Source: CAD feature listing. Evaluate the final solid. Frame: model axes, mm. Face numbers are marked on the shaded views. Round coordinates to 2 decimals unless told otherwise and drop trailing zeros. Order: outer loops, then holes, each group sorted by start corner. A loop starts at its lowest first (then second) coordinate and runs counter-clockwise, first axis right, second up. Notation, with made-up numbers: (76, -22.75) -> (86, -22.75) arc R20 cw to (86, 12.25) -> close; hole circle Ø3 at (87, 26). An arc over 180 degrees is marked (long way). Answer as CSV lines item,"result".
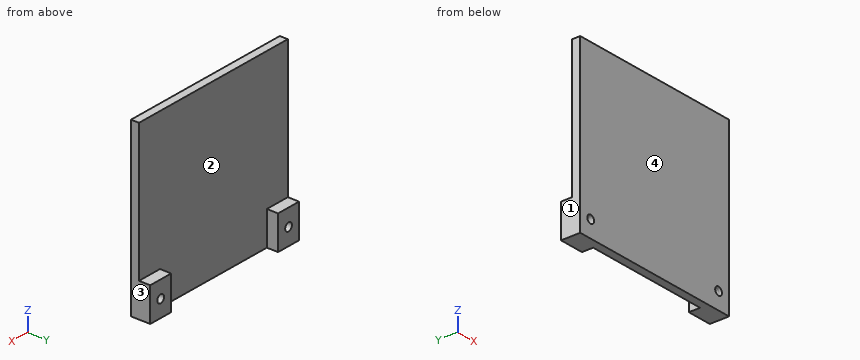
from build123d import *

# Parameters (mm, degrees)
SKETCH1_W                = 42.164
SKETCH1_H                = 40.64
SKETCH1_R                = 0.9525
BOSS_EXTRUDE1_DEPTH      = 1.27
BOSS_EXTRUDE1_DEPTH_BACK = 0.635
SKETCH1_4_W              = 5.9436
SKETCH1_4_H              = 8.001
SKETCH1_4_R              = 0.9525
BOSS_EXTRUDE2_DEPTH      = 3.937


with BuildPart() as part:
    # Sketch1 → Boss-Extrude1 (new body, two sides)
    with BuildSketch(Plane(origin=(0, 0, 0), x_dir=(1, 0, 0), z_dir=(0, 1, 0))) as boss_extrude1_sk:
        Rectangle(SKETCH1_W, SKETCH1_H)
        with Locations((18.1102, 16.3195)):
            Circle(SKETCH1_R, mode=Mode.SUBTRACT)
        with Locations((-18.1102, 16.3195)):
            Circle(SKETCH1_R, mode=Mode.SUBTRACT)
    extrude(amount=BOSS_EXTRUDE1_DEPTH)
    extrude(boss_extrude1_sk.sketch, amount=-BOSS_EXTRUDE1_DEPTH_BACK)

    # Sketch1_4 → Boss-Extrude2 (add)
    with BuildSketch(Plane(origin=(0, 0, 0), x_dir=(1, 0, 0), z_dir=(0, 1, 0))):
        with Locations((-18.1102, 16.3195)):
            Rectangle(SKETCH1_4_W, SKETCH1_4_H)
        with Locations((-18.1102, 16.3195)):
            Circle(SKETCH1_4_R, mode=Mode.SUBTRACT)
        with Locations((18.1102, 16.3195)):
            Rectangle(SKETCH1_4_W, SKETCH1_4_H)
        with Locations((18.1102, 16.3195)):
            Circle(SKETCH1_4_R, mode=Mode.SUBTRACT)
    extrude(amount=BOSS_EXTRUDE2_DEPTH)


solid = part.part
1. Section query B-B on x = -10. Return loops of the section in (y, z) (3 decimals), and give its area (3 significant figures).
Results below:
outline,"(-0.635, -20.32) -> (1.27, -20.32) -> (1.27, 20.32) -> (-0.635, 20.32) -> close"
area,"77.4 mm2"
2. Pin query (flat end, axial travel): pin 1 (3 mm diameter, centred on x = 11.5, z = -7, fed in from +Y); pin 2 (2 mm diameter, centred on x = 18.5, y = 2.5, fed in from +Z). Return the tip coordinate at first contact, or that it passes through.
Results below:
pin 1,"y = 1.27"
pin 2,"z = -12.32"
3. Section query A-A on y = 3.1. Return loops of the section in (x, z) (1 decimal).
Results below:
outline,"(-21.1, -20.3) -> (-15.1, -20.3) -> (-15.1, -12.3) -> (-21.1, -12.3) -> close; (15.1, -20.3) -> (21.1, -20.3) -> (21.1, -12.3) -> (15.1, -12.3) -> close; hole circle Ø1.9 at (-18.1, -16.3); hole circle Ø1.9 at (18.1, -16.3)"
4. Section query C-C on z = -11. Return loops of the section in (x, y) (3 decimals), and give its area (3 significant figures).
Results below:
outline,"(-21.082, -0.635) -> (21.082, -0.635) -> (21.082, 1.27) -> (-21.082, 1.27) -> close"
area,"80.3 mm2"
5. Line query: L1, parallel to X at y = 2.8, z = -17.5; L2, parallel to Y at x = -3, z = 18 (3 decimals). Output: solid intervals per line, ascending. Write a range as [from, to].
Results below:
L1,"[-21.08, -15.14], [15.14, 21.08]"
L2,"[-0.635, 1.27]"
6. Mould query, pull axis X, two halves, no side actions, for the marked faces 1, 2, 3 and 4. Classes: released by +X, released by -X, zero draft, split by the parting line, or undercut.
Results below:
face 1,"released by -X"
face 2,"undercut"
face 3,"released by +X"
face 4,"zero draft"
